from build123d import *

# Parameters (mm, degrees)
SKETCH_R      = 4
SKETCH_R_2    = 2.5
PAD_DEPTH     = 5
SKETCH001_R   = 10
SKETCH001_R_2 = 4
PAD001_DEPTH  = 5


with BuildPart() as part:
    # Sketch → Pad (new body)
    with BuildSketch(Plane.XY):
        with BuildLine():
            ThreePointArc((-2.3931586809, -9.7094176719), (0, -10), (2.3931586809, -9.7094176719))
            Line((2.3931586809, -9.7094176719), (21.5, -5))
            Line((21.5, -5), (21.5, 5))
            Line((21.5, 5), (2.3931586809, 9.7094176719))
            ThreePointArc((2.3931586809, 9.7094176719), (0, 10), (-2.3931586809, 9.7094176719))
            Line((-21.5, 5), (-2.3931586809, 9.7094176719))
            Line((-21.5, 5), (-21.5, -5))
            Line((-21.5, -5), (-2.3931586809, -9.7094176719))
        make_face()
        Circle(SKETCH_R, mode=Mode.SUBTRACT)
        with Locations((-16.5, 0)):
            Circle(SKETCH_R_2, mode=Mode.SUBTRACT)
        with Locations((16.5, 0)):
            Circle(SKETCH_R_2, mode=Mode.SUBTRACT)
    extrude(amount=PAD_DEPTH)

    # Sketch001 (on Face13 of Pad) → Pad001 (join)
    with BuildSketch(Plane.XY.offset(5)):
        Circle(SKETCH001_R)
        Circle(SKETCH001_R_2, mode=Mode.SUBTRACT)
    extrude(amount=PAD001_DEPTH)


solid = part.part
The model under review builds one solid part; all positions refer to its coordinate system, in mm. A direction names the side the tool comes from. Coordinates: 2 decimals unless noted, no trailing zeros. Loops run counter-clockwise (first coordinate to the right, second up) from the corner with the lowest first, then second, coordinate; pieces in that order, holes last.
(1) Consider section C-C, the plane z = 1.75. Give the boundary of the cut face in (x, y).
Determined:
outline: (-21.5, -5) - (-2.39, -9.71) arc R10 ccw to (2.39, -9.71) - (21.5, -5) - (21.5, 5) - (2.39, 9.71) arc R10 ccw to (-2.39, 9.71) - (-21.5, 5) - close; hole circle Ø5 at (-16.5, 0); hole circle Ø8 at (0, 0); hole circle Ø5 at (16.5, 0)
(2) Consider section A-A, the plane y = 0. Give the boundary of the cut face in (x, z).
Determined:
outline: (-21.5, 0) - (-19, 0) - (-19, 5) - (-21.5, 5) - close; (-14, 0) - (-4, 0) - (-4, 10) - (-10, 10) - (-10, 5) - (-14, 5) - close; (4, 0) - (14, 0) - (14, 5) - (10, 5) - (10, 10) - (4, 10) - close; (19, 0) - (21.5, 0) - (21.5, 5) - (19, 5) - close
(3) Tool access review of faces 1 (the flat face through (11.81, -7.39, 2.46)), 2 (the flat face through (-12, 0, 5)): name each direction out of +Z, -Z, +X, -X, +Y, -Y from which nothing blocks a thin tool from reaching the whole face with its end or side.
Determined:
face 1: +Z, -Z, +X, -Y
face 2: +Z, -X
(4) Insertion check: P1, Ø6, axis at x = 16.5, y = 0, coming from the +Z side; P2, Ø2, axis at x = 16.5, z = 1.5, coming from the -Y side; P3, Ø1, axis at x = 7, z = 1.5, coming from the +Y side. Each pin has a flat end and moves straight along its axis. Give the tip position at first contact, or say it passes through.
Determined:
P1: stops at z = 5
P2: stops at y = -6.48
P3: stops at y = 8.7
(5) Consider section D-D, the plane x = 5. Give the boundary of the cut face in (y, z), plus the area to 3 significant figures.
Determined:
outline: (-9.07, 0) - (9.07, 0) - (9.07, 5) - (8.66, 5) - (8.66, 10) - (-8.66, 10) - (-8.66, 5) - (-9.07, 5) - close
area: 177 mm2
(6) Wall thickness on L1, parallel to Z at x = -18, y = 5.25; L2, parallel to X at y = 2.25, z = 8; L3, parallel to Y at x = 0, z = 6.5: over which ranges is each line inside the solid? List them lowest first.
Determined:
L1: z = 0 to 5
L2: x = -9.74 to -3.31, 3.31 to 9.74
L3: y = -10 to -4, 4 to 10
(7) Consider section B-B, the plane x = 0. Give the boundary of the cut face in (y, z), plus the area to 3 significant figures.
Determined:
outline: (-10, 0) - (-4, 0) - (-4, 10) - (-10, 10) - close; (4, 0) - (10, 0) - (10, 10) - (4, 10) - close
area: 120 mm2
(8) Draft analysis for pull direction X (two halves, no side actions). For faces 3 (the flat face through (-0.3, -4.3, 0)), 4 (the flat face through (21.5, 0, 2)), 5 (the flat face through (-21.5, 0, 2)), 6 (the cylindrical face through (14, 0, 2)), state which applies: +X half, -X half, draft (parallel to the pull), parting line (faces both ways), or undercut.
Determined:
face 3: draft
face 4: +X half
face 5: -X half
face 6: undercut
